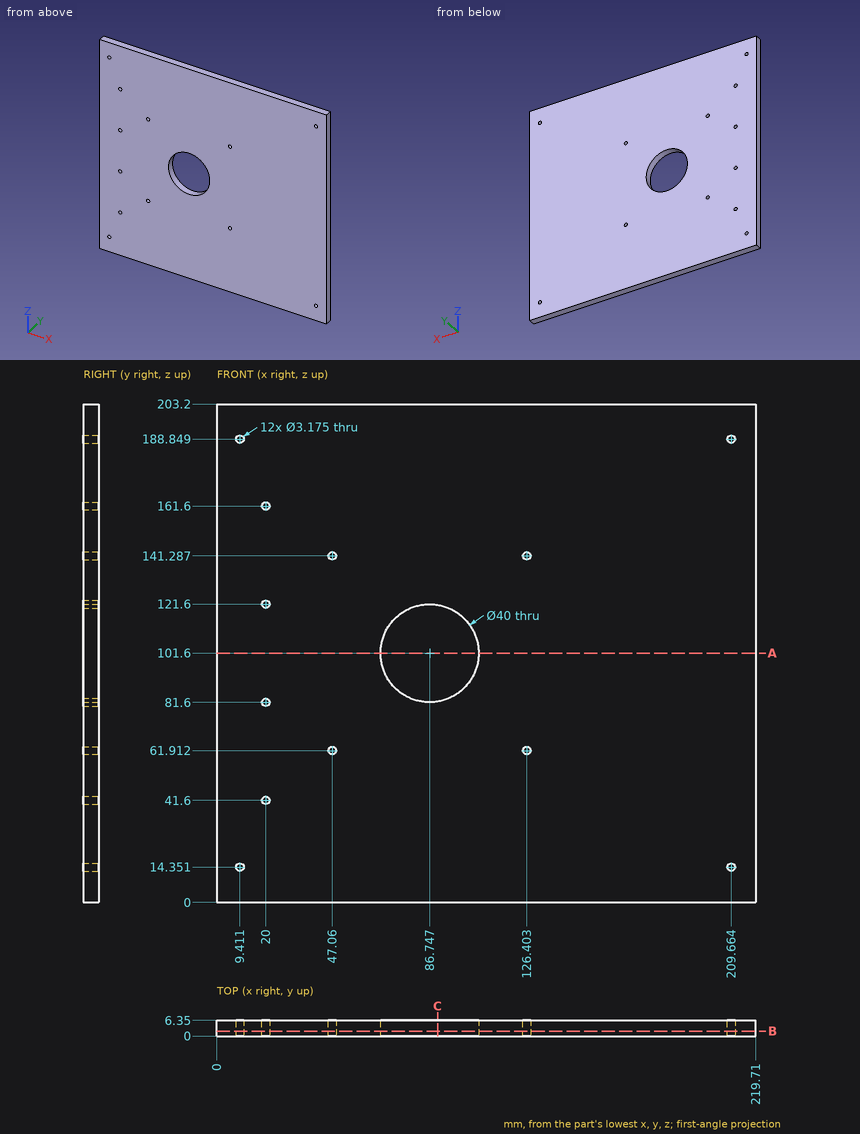
Could you check a few things on this drawing? It's one solid part, dimensions in mm from its lowest x, y, z. Round coordinates to 2 decimals unless told otherwise and drop trailing zeros. Order: outer loops, then holes, each group sorted by start corner. A loop starts at its lowest first (then second) coordinate and runs counter-clockwise, first axis right, second up. Notation, with made-up numbers: M -40,-0.75 L 14,-0.75 A34 cw 14,34.25 Z; hole C -2,3 d1. An arc over 180 degrees is marked long. Use a Markdown table: item, result.
1) If I drill on line 1 along Z through (x, y) = (20, 3); line 2 along X through (y, z) = (3.5, 41.6); line 3 along X through (y, z) = (3, 101.6), over which ranges is the centre line in solid material (lowest first)?
Geometry says:
| item | result |
|---|---|
| line 1 | z = 0 to 40.01, 43.19 to 80.01, 83.19 to 120.01, 123.19 to 160.01, 163.19 to 203.2 |
| line 2 | x = 0 to 18.41, 21.59 to 219.71 |
| line 3 | x = 0 to 66.75, 106.75 to 219.71 |
2) Imagine slicing it at B-B (y = 2). Give the number of separate pieces and of enclosed holes in the cut face, then the cut area to 3 significant figures.
Geometry says:
| item | result |
|---|---|
| separate pieces | 1 |
| enclosed holes | 13 |
| area | 43,300 mm² |
3) Imagine slicing it at A-A (z = 101.6). List the corners of the cut face in (x, y) for me.
Geometry says:
| item | result |
|---|---|
| outline | M 0,0 L 66.75,0 L 66.75,6.35 L 0,6.35 Z; M 106.75,0 L 219.71,0 L 219.71,6.35 L 106.75,6.35 Z |
4) I'm going to push a flat-ended pin straight in: P1, Ø2, axis at y = 3, z = 107, coming from the -X side. Where does the tip first touch, or does it pass through?
Geometry says:
| item | result |
|---|---|
| P1 | stops at x = 0 |
5) Imagine slicing it at C-C (x = 90). List the corners of the cut face in (y, z) for me, then the cut area to 3 significant figures.
Geometry says:
| item | result |
|---|---|
| outline | M 0,0 L 6.35,0 L 6.35,81.87 L 0,81.87 Z; M 0,121.33 L 6.35,121.33 L 6.35,203.2 L 0,203.2 Z |
| area | 1,040 mm² |
